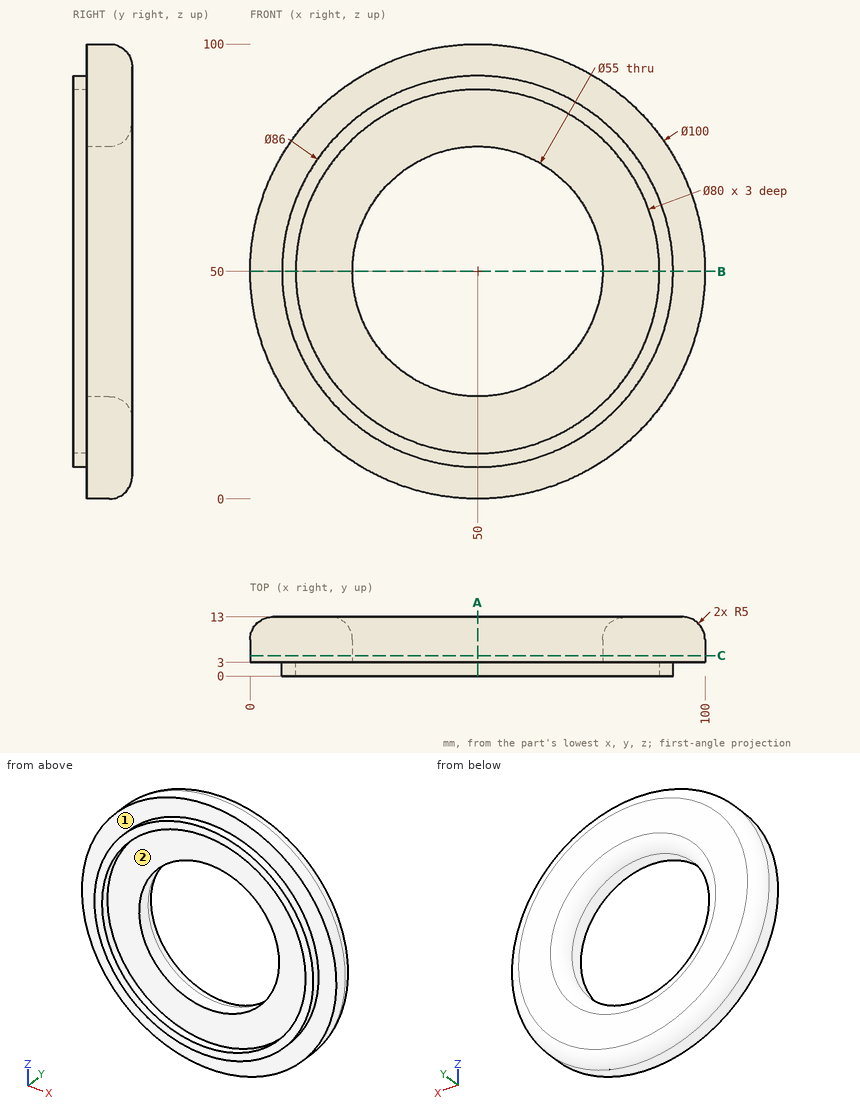
The drawing under review shows one solid part. Ordinate dimensions are in mm from its lowest x, y, z. Give positions to 0.01 mm unless a question says otherwise; leave off trailing zeros. Loops run counter-clockwise (first coordinate to the right, second up) from the corner with the lowest first, then second, coordinate; pieces in that order, holes last. Notation, with made-up numbers: M -13,18.5 L 15,18.5 A27 ccw 15,37.5 Z; hole C -3.5,45 d5. An arc over 180 degrees is marked long. One line per question, with ' | ' between items. Start each with the question number.
1. Add section B-B (z = 50). Write out the cut boundary in (x, y), plus the area to 3 significant figures.
2. To check wall thickness, follow L1, parallel to X at y = 1.2, z = 50; L2, parallel to Y at x = 63.5, z = 7; L3, parallel to Z at x = 68.5, y = 10. State the ranges of each line that lie inside material, in increasing order.
3. Add section C-C (y = 4.5). Write out the cut boundary in (x, z), plus the area to 3 significant figures.
4. The part is to be moulded in two halves that separate along X. For the marked faces 1 and 2, say which applies: released by +X, released by -X, zero draft, split by the parting line, or undercut.
5. Insertion check: P1, Ø1, axis at y = 11.5, z = 29.5, coming from the -X side; P2, Ø4, axis at x = 64, z = 24, coming from the -Y side; P3, Ø6, axis at x = 76, y = 7, coming from the -Z side. Each pin has a flat end and moves straight along its axis. Give the tip position at first contact, or say it passes through.
6. Add section A-A (x = 50). Write out the cut boundary in (y, z).
Worked out:
1) outline: M 0,3 L 7,3 L 7,0 L 10,0 L 10,3 L 22.5,3 L 22.5,8 A5 ccw 17.5,13 L 5,13 A5 ccw 0,8 Z; M 77.5,3 L 90,3 L 90,0 L 93,0 L 93,3 L 100,3 L 100,8 A5 ccw 95,13 L 82.5,13 A5 ccw 77.5,8 Z | area: 447 mm²
2) L1: x = 7 to 10, 90 to 93 | L2: y = 3 to 13 | L3: z = 4 to 29.09, 70.91 to 96
3) outline: C 50,50 d100; hole C 50,50 d55 | area: 5,480 mm²
4) face 1: zero draft | face 2: undercut
5) P1: stops at x = 5.44 | P2: stops at y = 3 | P3: stops at z = 5.6
6) outline: M 0,7 L 3,7 L 3,0 L 8,0 A5 ccw 13,5 L 13,17.5 A5 ccw 8,22.5 L 3,22.5 L 3,10 L 0,10 Z; M 0,90 L 3,90 L 3,77.5 L 8,77.5 A5 ccw 13,82.5 L 13,95 A5 ccw 8,100 L 3,100 L 3,93 L 0,93 Z
